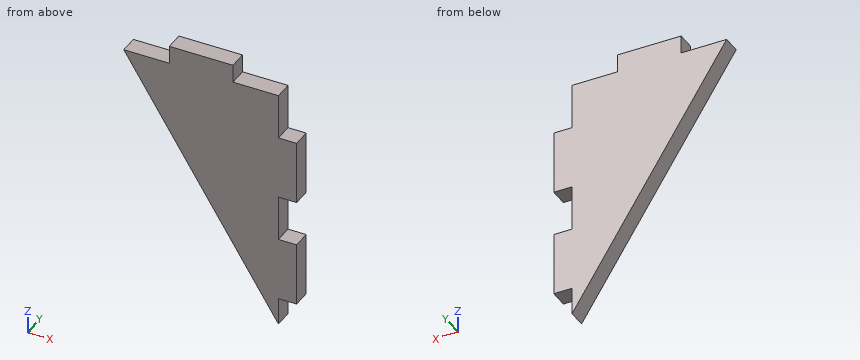
```python
from build123d import *

# Parameters (mm, degrees)
SKETCH1_W           = 7
SKETCH1_H           = 2
SKETCH1_W_2         = 2
SKETCH1_H_2         = 7
BOSS_EXTRUDE1_DEPTH = 2


with BuildPart() as part:
    # Sketch1 → Boss-Extrude1 (new body)
    with BuildSketch(Plane(origin=(0, 0, 0), x_dir=(1, 0, 0), z_dir=(0, 1, 0))):
        Polygon((0, 27), (0, 0), (-17, 0), align=None)
        with Locations((-8.5, -1)):
            Rectangle(SKETCH1_W, SKETCH1_H)
        with Locations((1, 8.5)):
            Rectangle(SKETCH1_W_2, SKETCH1_H_2)
        with Locations((1, 20.5)):
            Rectangle(SKETCH1_W_2, SKETCH1_H_2)
    extrude(amount=BOSS_EXTRUDE1_DEPTH)


solid = part.part
```
Build history of the part. All positions in model axes, mm. Give positions to 0.01 mm unless a question says otherwise; leave off trailing zeros. Loops run counter-clockwise (first coordinate to the right, second up) from the corner with the lowest first, then second, coordinate; pieces in that order, holes last. Notation, with made-up numbers: (72.25, -32) -> (89.25, -32) arc R28 ccw to (89.25, -14) -> close; hole circle Ø1 at (47.5, -13.75). An arc over 180 degrees is marked (long way). One line per question, with ' | ' between items. Start each with the question number.
1) Cut at C-C (x = -3.75). Give the cut face in (y, z), plus the area to 3 significant figures.
2) Pin check, flat tips, straight feed: pin 1 (1 mm diameter, centred on x = 1, y = 1.5, fed in from +Z); pin 2 (1 mm diameter, centred on x = -15, z = -5.5, fed in from +Y); pin 3 (1 mm diameter, centred on y = 1, z = -14.5, fed in from +X). Stop position of each tip, or through.
3) Probe L1, parallel to X at y = 0.35, z = -16; L2, parallel to X at y = 1.7, z = -14.75; L3, parallel to Z at x = -11, y = 0.1. List the from-to ranges inside material, lowest first.
4) Cut at A-A (y = 1.35). Give the cut face in (x, z), plus the area to 4 significant figures.
5) Cut at B-B (z = -20.25). Give the cut face in (x, y).
Return value:
1) outline: (0, -21.04) -> (2, -21.04) -> (2, 0) -> (0, 0) -> close | area: 42.1 mm^2
2) pin 1: z = -5 | pin 2: through | pin 3: x = 0
3) L1: -6.93 to 0 | L2: -7.71 to 0 | L3: -9.53 to 2
4) outline: (-17, 0) -> (0, -27) -> (0, -24) -> (2, -24) -> (2, -17) -> (0, -17) -> (0, -12) -> (2, -12) -> (2, -5) -> (0, -5) -> (0, 0) -> (-5, 0) -> (-5, 2) -> (-12, 2) -> (-12, 0) -> close | area: 271.5 mm^2
5) outline: (-4.25, 0) -> (2, 0) -> (2, 2) -> (-4.25, 2) -> close
